Job drawing, mm, ordinate dimensions from the low corner. One solid piece. A direction names the side the tool comes from. Round coordinates to 2 decimals unless told otherwise and drop trailing zeros. Write each loop counter-clockwise with the first axis right and the second up, starting at its lowest first coordinate (ties: lowest second). Pieces come first, ordered by that corner, then holes.
1) Which spindle directions (+Z, -Z, +X, -X, +Y, -Y) get a long thin tool onto all of the face, cutting with end or side? Do the marked faces 1, 2 and 3. Say none if no direction does.
2) Saw through at C-C on y = 182. Write the cut outline in (x, z), and give its area (3 significant figures).
3) Drill centre lines: L1, parallel to Y at x = 558.8, z = 53.75; L2, parallel to Y at x = 157.5, z = 45; L3, parallel to Z at x = 420, y = 157. Where is each one in solid material? Low to high.
4) Flat gauge pins, fed straight in: pin 1 (6 mm diameter, centred on x = 164.5, y = 269, fed in from +Z); pin 2 (12 mm diameter, centred on x = 116.5, z = 17.5, fed in from +Y); pin 3 (24.5 mm diameter, centred on x = 377.5, z = 35.5, fed in from -Y). Where does each tip first touch, or does it go through?
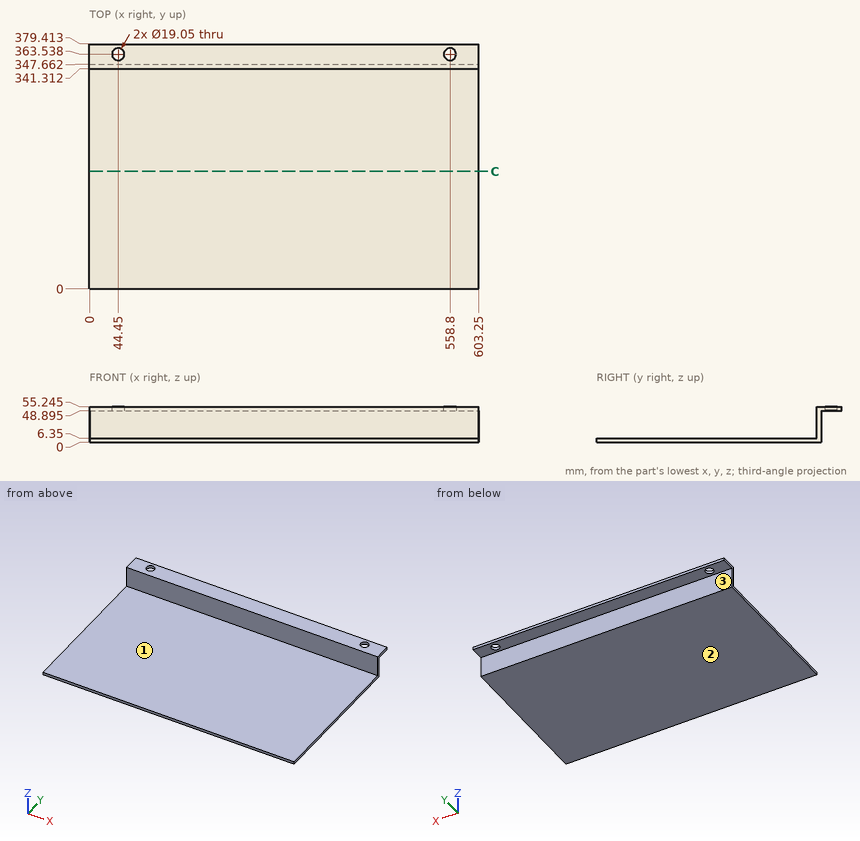
Completed:
1. face 1: +Z, +X, -X, -Y
1. face 2: -Z, +X, -X, +Y, -Y
1. face 3: -Z, +X, -X, +Y
2. outline: (0, 0) - (603.25, 0) - (603.25, 6.35) - (0, 6.35) - close
2. area: 3,830 mm2
3. L1: y = 341.31 to 354.01, 373.06 to 379.41
3. L2: y = 341.31 to 347.66
3. L3: z = 0 to 6.35
4. pin 1: stops at z = 6.35
4. pin 2: stops at y = 347.66
4. pin 3: stops at y = 341.31
